Can you work these out from the drawing? Everything is in mm from the part's minimum corner. Coordinates: 2 decimals unless noted, no trailing zeros. Write each loop counter-clockwise with the first axis right and the second up, starting at its lowest first coordinate (ties: lowest second). Pieces come first, ordered by that corner, then holes. Notation, with made-up numbers: (49, 72.5) -> (79, 72.5) arc R16 ccw to (79, 88.5) -> close; hole circle Ø6 at (40, 32.5). An arc over 180 degrees is marked (long way). Use a Markdown table: item, result. Add a question column.
Item 1: If I drill on line 1 along Z through (x, y) = (260.35, 9.75) (3 decimals); line 2 along X through (y, z) = (9, 24.5); line 3 along X through (y, z) = (11.25, 45), over which ranges is the centre line in solid material (lowest first)? Write a range as from..to.
Item 2: Imagine slicing it at B-B, the plane z = 11. Write out the boundary of the cut face in (x, y), and give its area (3 significant figures).
Item 3: Imagine slicing it at C-C, the plane z = 55. Write out the boundary of the cut face in (x, y), and give its area (3 significant figures).
Item 4: Imagine slicing it at A-A, the plane y = 11.5. Write out the boundary of the cut face in (x, z) (3 decimals).
Item 5: Will these pins go through, and if not, where does the flat tip stop? pin 1 Ø4 at (x, y) = (81.5, 2) entering from -Z; pin 2 Ø3 at (y, z) = (12, 32) entering from -X; pin 3 Ø1.5 at (y, z) = (13.5, 13) entering from +X; pin 4 Ø3 at (y, z) = (5.5, 31) entering from +X.
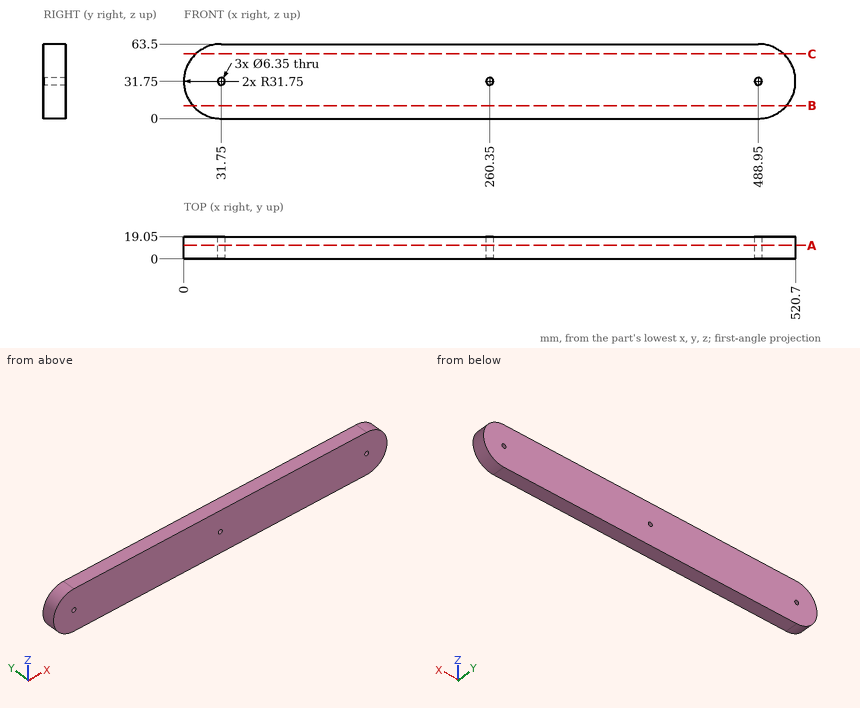
Ans:
| question | item | result |
|---|---|---|
| 1 | line 1 | z = 0..28.575, 34.925..63.5 |
| 1 | line 2 | x = 0.84..519.86 |
| 1 | line 3 | x = 2.9..517.8 |
| 2 | outline | (7.72, 0) -> (512.98, 0) -> (512.98, 19.05) -> (7.72, 19.05) -> close |
| 2 | area | 9,630 mm^2 |
| 3 | outline | (10.13, 0) -> (510.57, 0) -> (510.57, 19.05) -> (10.13, 19.05) -> close |
| 3 | area | 9,530 mm^2 |
| 4 | outline | (31.75, 0) -> (488.95, 0) arc R31.75 ccw to (488.95, 63.5) -> (31.75, 63.5) arc R31.75 ccw to start; hole circle Ø6.35 at (31.75, 31.75); hole circle Ø6.35 at (260.35, 31.75); hole circle Ø6.35 at (488.95, 31.75) |
| 5 | pin 1 | stops at z = 0 |
| 5 | pin 2 | stops at x = 0 |
| 5 | pin 3 | stops at x = 515.1 |
| 5 | pin 4 | stops at x = 520.7 |
